Geometry check sheet. Reference: the model listing, model coordinates, mm. Round coordinates to 2 decimals unless told otherwise and drop trailing zeros. Order: outer loops, then holes, each group sorted by start corner. A loop starts at its lowest first (then second) coordinate and runs counter-clockwise, first axis right, second up. Notation, with made-up numbers: M 58.25,-28.5 L 100.25,-28.5 A9 cw 100.25,-15.5 Z; hole C -31,22 d11. An arc over 180 degrees is marked long. Return JSON: item names as keys, results as strings. Group by question number.
```python
from build123d import *

# Parameters (mm, degrees)
ESQUISSE1_W             = 140
ESQUISSE1_H             = 87
ESQUISSE1_R             = 2.75
ESQUISSE1_R_2           = 1.6
ESQUISSE1_R_3           = 12.5
BOSS_EXTRU_1_DEPTH      = 2
ESQUISSE2_W             = 30
ESQUISSE2_H             = 50
ENL_V_MAT_EXTRU_1_DEPTH = 10


with BuildPart() as part:
    # Esquisse1 → Boss.-Extru.1 (new body)
    with BuildSketch(Plane(origin=(0, 0, 0), x_dir=(1, 0, 0), z_dir=(0, 1, 0))):
        Rectangle(ESQUISSE1_W, ESQUISSE1_H)
        with Locations((-60, -23.5)):
            Circle(ESQUISSE1_R, mode=Mode.SUBTRACT)
        with Locations((-28, -23.5)):
            Circle(ESQUISSE1_R, mode=Mode.SUBTRACT)
        with Locations((28, -23.5)):
            Circle(ESQUISSE1_R, mode=Mode.SUBTRACT)
        with Locations((60, -23.5)):
            Circle(ESQUISSE1_R, mode=Mode.SUBTRACT)
        with Locations((-15.5, 30.5)):
            Circle(ESQUISSE1_R_2, mode=Mode.SUBTRACT)
        with Locations((15.5, 30.5)):
            Circle(ESQUISSE1_R_2, mode=Mode.SUBTRACT)
        with Locations((15.5, -0.5)):
            Circle(ESQUISSE1_R_2, mode=Mode.SUBTRACT)
        with Locations((-15.5, -0.5)):
            Circle(ESQUISSE1_R_2, mode=Mode.SUBTRACT)
        with Locations((0, 15)):
            Circle(ESQUISSE1_R_3, mode=Mode.SUBTRACT)
    extrude(amount=BOSS_EXTRU_1_DEPTH)

    # Esquisse2 → Enlèv. mat.-Extru.1 (cut)
    with BuildSketch(Plane(origin=(0, 2, 0), x_dir=(1, 0, 0), z_dir=(0, 1, 0))):
        with Locations((-55, 18.5)):
            Rectangle(ESQUISSE2_W, ESQUISSE2_H)
        with Locations((55, 18.5)):
            Rectangle(ESQUISSE2_W, ESQUISSE2_H)
    extrude(amount=-ENL_V_MAT_EXTRU_1_DEPTH, mode=Mode.SUBTRACT)


solid = part.part
```
Q1. Section check B-B on y = 1.65. Count the separate pieces of the cut face and the enclosed holes in it, plus the area to 3 significant figures.
Q2. Section check D-D on z = -15. Record the cut outline in (x, y).
Q3. Release check for a two-part mould opening along X. For faces 1 (the face through (-17.1, 0.99, -30.57)), 2 (the face through (-1, 0, 9)) record: +X half, -X half, draft (parallel to the pull), parting line (faces both ways), or undercut.
Q4. Depth check by flat-ended pin: pin 1 Ø4.5 at (x, z) = (-28, 23.5) entering from -Y; pin 2 Ø1 at (x, y) = (47.5, 0.5) entering from -Z; pin 3 Ø1 at (y, z) = (1, -30.5) entering from -X. Enter the tip coordinate at first touch or a pass-through.
Q5. Section check C-C on x = -28. Record the cut outline in (y, z), plus the area to 3 significant figures.
Q6. Material ranges on line 1 along X through (y, z) = (1.15, 0.5); line 2 along Z through (x, y) = (-15.5, 1.15); line 3 along X through (y, z) = (0.6, 23.5), recorded low to high.
Q7. Section check A-A on z = -30.5. Record the cut outline in (x, y), plus the area to 3 significant figures.
Geometry check:
{
 "1": {"separate pieces": "1", "enclosed holes": "9", "area": "8,560 mm^2"},
 "2": {"outline": "M -40,0 L -12.5,0 L -12.5,2 L -40,2 Z; M 12.5,0 L 40,0 L 40,2 L 12.5,2 Z"},
 "3": {"face 1": "undercut", "face 2": "draft"},
 "4": {"pin 1": "passes through", "pin 2": "stops at z = 6.5", "pin 3": "stops at x = -40"},
 "5": {"outline": "M 0,-43.5 L 2,-43.5 L 2,20.75 L 0,20.75 Z; M 0,26.25 L 2,26.25 L 2,43.5 L 0,43.5 Z", "area": "163 mm^2"},
 "6": {"line 1": "x = -40 to -17.1, -13.9 to 13.9, 17.1 to 40", "line 2": "z = -43.5 to -32.1, -28.9 to -1.1, 2.1 to 43.5", "line 3": "x = -70 to -62.75, -57.25 to -30.75, -25.25 to 25.25, 30.75 to 57.25, 62.75 to 70"},
 "7": {"outline": "M -40,0 L -17.1,0 L -17.1,2 L -40,2 Z; M -13.9,0 L 13.9,0 L 13.9,2 L -13.9,2 Z; M 17.1,0 L 40,0 L 40,2 L 17.1,2 Z", "area": "147 mm^2"}
}
